Autodesk Inventor part; units mm, degrees
ref_plane "YZ Plane" through (0, 0, 0) normal (1, 0, 0) x (0, 1, 0)
ref_plane "XZ Plane" through (0, 0, 0) normal (0, 1, 0) x (-1, 0, 0)
ref_plane "XY Plane" through (0, 0, 0) normal (0, 0, 1) x (1, 0, 0)
sketch "Sketch1" plane through (0, 0, 0) normal (0, 1, 0) x (-1, 0, 0)
  line L0 (0, 0) -> (0, -80)
  line L1 (50, -90) -> (0, -80)
  line L2 (0, -70) -> (-10.5, -70)
  line L3 (-10.5, -70) -> (-10.5, -15.1)
  line L4 (-10.5, -15.1) -> (0, -15.1)
  line L5 (0, -15.1) -> (-4, -15.1)
  line L6 (-4, -15.1) -> (-4, -70) construction
  line L7 (50, -90) -> (50, -40)
  line L8 (50, -40) -> (0, 0)
  dimension "d0" = 80
  dimension "d1" = 50
  dimension "d5" = 10
  dimension "d6" = 54.9
  dimension "d9" = 4
extrude "Extrusion1" add sketch "Sketch1" along normal mid plane 3
properties part number "Stateczniki"
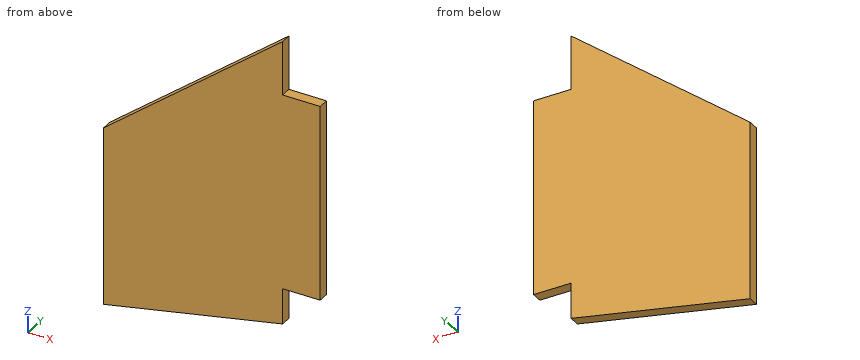
CAD build for the part. Positions are in the model's coordinates, mm. Round coordinates to 2 decimals unless told otherwise and drop trailing zeros. Order: outer loops, then holes, each group sorted by start corner. A loop starts at its lowest first (then second) coordinate and runs counter-clockwise, first axis right, second up. Notation, with made-up numbers: (-22.75, -10.5) - (-4.75, -10.5) arc R33 cw to (-4.75, 19.5) - close; hole circle Ø5 at (0.5, 57.5). An arc over 180 degrees is marked (long way). Return JSON: item names as keys, results as strings.
(1) Wall check: probe 1 along Z at (x, y) = (7.5, -0.9); probe 2 along X at (y, z) = (-1, -79); probe 3 along Z at (x, y) = (-19.5, 0.95). Give the ranges that are in metal, low to high. Write a range as from..to.
Answer key:
{"probe 1": "z = -70..-15.1", "probe 2": "x = -50..0", "probe 3": "z = -83.9..-15.6"}
(2) Cut at B-B (x = -28). Give the cut face in (y, z), then the cut area to 3 significant figures.
Answer key:
{"outline": "(-1.5, -85.6) - (1.5, -85.6) - (1.5, -22.4) - (-1.5, -22.4) - close", "area": "190 mm^2"}
(3) Pin check, flat tips, straight feed: pin 1 Ø0.9 at (x, y) = (6.5, -0.5) entering from +Z; pin 2 Ø1 at (x, y) = (-5, -0.5) entering from +Z; pin 3 Ø1.5 at (x, y) = (2.5, 0.5) entering from -Z. Stop position of each tip, or through.
Answer key:
{"pin 1": "stops at z = -15.1", "pin 2": "stops at z = -3.6", "pin 3": "stops at z = -70"}
(4) Cut at A-A (y = -0.3). Give the cut face in (x, z), then the cut area to 3 significant figures.
Answer key:
{"outline": "(-50, -90) - (0, -80) - (0, -70) - (10.5, -70) - (10.5, -15.1) - (0, -15.1) - (0, 0) - (-50, -40) - close", "area": "3,830 mm^2"}
(5) Cut at C-C (z = -36). Give the cut face in (x, y), then the cut area to 4 significant figures.
Answer key:
{"outline": "(-45, -1.5) - (10.5, -1.5) - (10.5, 1.5) - (-45, 1.5) - close", "area": "166.5 mm^2"}
